Geometry check sheet. Reference: the model listing, model coordinates, mm. A direction names the side the tool comes from. Round coordinates to 2 decimals unless told otherwise and drop trailing zeros. Order: outer loops, then holes, each group sorted by start corner. A loop starts at its lowest first (then second) coordinate and runs counter-clockwise, first axis right, second up.
(1) Draft check along X on faces 1 (the face through (-5, -10, 73)), 2 (the face through (105, -8, 70)), 3 (the face through (-15, -8, 70)). Enter one of: pulls with the +X half, pulls with the -X half, needs draft (parallel to the pull), parting line crosses it, or undercut.
(2) Cross-section at A-A on z = 63.25. Enter the section's corners in (x, y).
(3) Thickness scan on L1, parallel to Y at x = -7.5, z = 78; L2, parallel to X at y = -10.25, z = 77; L3, parallel to X at y = -8.5, z = 68.75. Record the ranges inside material, lowest first.
(4) Set-up check for faces 4 (the face through (44, -7, 79.5)), 5 (the face through (-5, -12.4, 76.3)): record each of +Z, -Z, +X, -X, +Y, -Y from which the full face is reachable in a straight line by a thin tool's end or side.
(5) Cross-section at C-C on y = -7.5. Enter the section's corners in (x, z).
(6) Cross-section at B-B on x = -7.5. Enter the section's corners in (y, z), and give its area (3 significant figures).
(7) Gauge pin test, flat ends, axial feed: P1, Ø7.5, axis at x = -7.5, y = -7.5, coming from the +Z side; P2, Ø5, axis at x = 97.5, y = -7.5, coming from the +Z side. Record the tip position at first contact, or that the pin passes through.
(8) Cross-section at D-D on z = 77.75. Enter the section's corners in (x, y).
from build123d import *

# Parameters (mm, degrees)
F1_DEPTH         = 15
F2_W             = 74
F2_H             = 5
F3_DEPTH         = 15
F4_R             = 4.99999
F5_R             = 8
F8_D             = 7
F11_D            = 5
F11_DEPTH        = 20
F11_TIP          = 1.5021515476
F11_ON_F10_D     = 5
F11_ON_F10_DEPTH = 20
F11_ON_F10_TIP   = 1.5021515476
F12_W            = 105
F12_H            = 15
F12_W_2          = 15
F12_R            = 2.5
F13_DEPTH        = 18
F16_D            = 6.5
F16_CBORE_D      = 11
F16_CBORE_DEPTH  = 6.5


# Not quite as in the source:
# - a fillet or chamfer is up to 0.001 mm smaller than in the source, because OpenCascade refuses the exact size
# - a feature of the source that left no trace in its solid (it failed there, or was rolled back) is left out


with BuildPart() as f1:
    # F0 (on Front) → F1 (new body)
    with BuildSketch(Plane.XZ):
        Polygon((90, 0), (0, 0), (0, 61.5), (-15, 61.5), (-15, -15), (105, -15), (105, 61.5), (90, 61.5), align=None)
    extrude(amount=F1_DEPTH)

    # F2 (on face) → F3 (join, through all)
    with BuildSketch(Plane.XZ.offset(15)):
        with Locations((45, -17.5)):
            Rectangle(F2_W, F2_H)
    extrude(amount=-F3_DEPTH)

    # F4 (radius 5 in the source; OpenCascade refuses exactly that, so slightly less here)
    f4_edges = [f1.edges().sort_by_distance(p)[0] for p in [
        (0, -7.5, 0),
        (90, -7.5, 0),
        (8, -7.5, -15),
        (82, -7.5, -15),
    ]]
    fillet(f4_edges, radius=F4_R)

    # F5
    f5_edges = [f1.edges().sort_by_distance(p)[0] for p in [
        (-15, -7.5, -15),
        (105, -7.5, -15),
    ]]
    fillet(f5_edges, radius=F5_R)

    # F8 (through all)
    with Locations(Plane.XZ.offset(15)):
        with Locations((19.6, -10), (70.4, -10)):
            Hole(F8_D / 2)

    # F11
    with Locations(Plane.XY.offset(61.5)):
        with Locations((-7.5, -7.5)):
            Hole(F11_D / 2, depth=F11_DEPTH)
            with Locations((0, 0, -(F11_DEPTH + F11_TIP / 2))):  # 118° drill point
                Cone(0, F11_D / 2, F11_TIP, mode=Mode.SUBTRACT)

    # F11 on F10
    with Locations(Plane.XY.offset(61.5)):
        with Locations((97.5, -7.5)):
            Hole(F11_ON_F10_D / 2, depth=F11_ON_F10_DEPTH)
            with Locations((0, 0, -(F11_ON_F10_DEPTH + F11_ON_F10_TIP / 2))):  # 118° drill point
                Cone(0, F11_ON_F10_D / 2, F11_ON_F10_TIP, mode=Mode.SUBTRACT)


with BuildPart() as f13:
    # F12 (on face) → F13 (new body)
    with BuildSketch(Plane.XY.offset(61.5)):
        with Locations((52.5, -7.5)):
            Rectangle(F12_W, F12_H)
        with Locations((-7.5, -7.5)):
            Rectangle(F12_W_2, F12_H)
        with Locations((-7.5, -7.5)):
            Circle(F12_R, mode=Mode.SUBTRACT)
    extrude(amount=F13_DEPTH)

    # F16 (through all)
    with Locations(Plane.XY.offset(79.5)):
        with Locations((-7.5, -7.5), (97.5, -7.5)):
            CounterBoreHole(F16_D / 2, F16_CBORE_D / 2, F16_CBORE_DEPTH)


solid = f13.part
Found:
1. face 1: undercut
1. face 2: pulls with the +X half
1. face 3: pulls with the -X half
2. outline: (-15, -15) - (105, -15) - (105, 0) - (-15, 0) - close; hole circle Ø6.5 at (-7.5, -7.5); hole circle Ø6.5 at (97.5, -7.5)
3. L1: y = -15 to -13, -2 to 0
3. L2: x = -15 to -12.26, -2.74 to 92.74, 102.26 to 105
3. L3: x = -15 to -10.59, -4.41 to 94.41, 100.59 to 105
4. face 4: +Z, +X, -X, +Y, -Y
4. face 5: +Z
5. outline: (-15, 61.5) - (-10.75, 61.5) - (-10.75, 73) - (-13, 73) - (-13, 79.5) - (-15, 79.5) - close; (-4.25, 61.5) - (94.25, 61.5) - (94.25, 73) - (92, 73) - (92, 79.5) - (-2, 79.5) - (-2, 73) - (-4.25, 73) - close; (100.75, 61.5) - (105, 61.5) - (105, 79.5) - (103, 79.5) - (103, 73) - (100.75, 73) - close
6. outline: (-15, 61.5) - (-10.75, 61.5) - (-10.75, 73) - (-13, 73) - (-13, 79.5) - (-15, 79.5) - close; (-4.25, 61.5) - (0, 61.5) - (0, 79.5) - (-2, 79.5) - (-2, 73) - (-4.25, 73) - close
6. area: 124 mm2
7. P1: stops at z = 73
7. P2: passes through
8. outline: (-15, -15) - (105, -15) - (105, 0) - (-15, 0) - close; hole circle Ø11 at (-7.5, -7.5); hole circle Ø11 at (97.5, -7.5)
